For this review, take the finished solid that the model builds, in its own axes (mm). Face numbers are marked on the shaded views. Coordinates: 2 decimals unless noted, no trailing zeros. Loops run counter-clockwise (first coordinate to the right, second up) from the corner with the lowest first, then second, coordinate; pieces in that order, holes last. Notation, with made-up numbers: (67, 68) -> (107, 68) arc R22 cw to (107, 88) -> close; hole circle Ø2 at (-19, 80). An arc over 180 degrees is marked (long way). Answer in a Markdown table with one row per item.
from build123d import *

# Parameters (mm, degrees)
F1_DEPTH = 7.2


with BuildPart() as f1:
    # F0 (on Top) → F1 (new body)
    with BuildSketch(Plane.XY):
        with BuildLine():
            ThreePointArc((-22.7073595632, -1.902869179), (-37.6721050646, -21.75), (-13.0016128307, -18.7137156451))
            ThreePointArc((-13.0016128307, -18.7137156451), (-14.4400957969, -19.1971358452), (-15.9320338179, -19.4747133584))
            ThreePointArc((-15.9320338179, -19.4747133584), (-35.5070415552, -20.5), (-24.8316134088, -4.060189341))
            ThreePointArc((-24.8316134088, -4.060189341), (-23.8452552203, -2.9069218706), (-22.7073595632, -1.902869179))
        make_face()
        with BuildLine():
            ThreePointArc((-6.75, -11.6913429511), (-9.545941546, -9.545941546), (-11.6913429511, -6.75))
            Line((-11.6913429511, -6.75), (-14.2894191624, -8.25))
            ThreePointArc((-14.2894191624, -8.25), (-12.9407634586, -11.5059428911), (-12.4807621135, -15))
            ThreePointArc((-12.4807621135, -15), (-12.6116088995, -16.8750312906), (-13.0016128307, -18.7137156451))
            ThreePointArc((-13.0016128307, -18.7137156451), (-9.0739087263, -15.9164124969), (-6.75, -11.6913429511))
        make_face()
        with BuildLine():
            Line((-14.2894191624, -8.25), (-11.6913429511, -6.75))
            ThreePointArc((-11.6913429511, -6.75), (-13.0399986549, -3.4940571089), (-13.5, 0))
            Line((-13.5, 0), (-18.7587036207, 0))
            ThreePointArc((-18.7587036207, 0), (-20.8303192969, -0.7495522538), (-22.7073595632, -1.902869179))
            ThreePointArc((-22.7073595632, -1.902869179), (-17.8531905577, -4.2207337632), (-14.2894191624, -8.25))
        make_face()
        with BuildLine():
            Line((-16.4544826719, -9.5), (-14.2894191624, -8.25))
            ThreePointArc((-14.2894191624, -8.25), (-17.8531905577, -4.2207337632), (-22.7073595632, -1.902869179))
            ThreePointArc((-22.7073595632, -1.902869179), (-23.8452552203, -2.9069218706), (-24.8316134088, -4.060189341))
            ThreePointArc((-24.8316134088, -4.060189341), (-19.9900128675, -5.7744418342), (-16.4544826719, -9.5))
        make_face()
        with BuildLine():
            ThreePointArc((-12.4807621135, -15), (-12.9407634586, -11.5059428911), (-14.2894191624, -8.25))
            Line((-14.2894191624, -8.25), (-16.4544826719, -9.5))
            ThreePointArc((-16.4544826719, -9.5), (-15.3555780244, -12.1529905039), (-14.9807621135, -15))
            ThreePointArc((-14.9807621135, -15), (-15.221207958, -17.2873553231), (-15.9320338179, -19.4747133584))
            ThreePointArc((-15.9320338179, -19.4747133584), (-14.4400957969, -19.1971358452), (-13.0016128307, -18.7137156451))
            ThreePointArc((-13.0016128307, -18.7137156451), (-12.6116088995, -16.8750312906), (-12.4807621135, -15))
        make_face()
        with BuildLine():
            Line((16.4544826719, -9.5), (14.2894191624, -8.25))
            ThreePointArc((14.2894191624, -8.25), (12.5818579404, -13.35094968), (13.0016128307, -18.7137156451))
            ThreePointArc((13.0016128307, -18.7137156451), (14.4400957969, -19.1971358452), (15.9320338179, -19.4747133584))
            ThreePointArc((15.9320338179, -19.4747133584), (14.9958197548, -14.4246380482), (16.4544826719, -9.5))
        make_face()
        with BuildLine():
            Line((14.2894191624, -8.25), (11.6913429511, -6.75))
            ThreePointArc((11.6913429511, -6.75), (9.545941546, -9.545941546), (6.75, -11.6913429511))
            ThreePointArc((6.75, -11.6913429511), (9.0739087263, -15.9164124969), (13.0016128307, -18.7137156451))
            ThreePointArc((13.0016128307, -18.7137156451), (12.5818579404, -13.35094968), (14.2894191624, -8.25))
        make_face()
        with BuildLine():
            Line((18.7587036207, 0), (13.5, 0))
            ThreePointArc((13.5, 0), (13.0399986549, -3.4940571089), (11.6913429511, -6.75))
            Line((11.6913429511, -6.75), (14.2894191624, -8.25))
            ThreePointArc((14.2894191624, -8.25), (17.8531905577, -4.2207337632), (22.7073595632, -1.902869179))
            ThreePointArc((22.7073595632, -1.902869179), (20.8303192969, -0.7495522538), (18.7587036207, 0))
        make_face()
        with BuildLine():
            ThreePointArc((39.4807621135, -15), (34.2891634511, -4.3594893349), (22.7073595632, -1.902869179))
            ThreePointArc((22.7073595632, -1.902869179), (23.8452552203, -2.9069218706), (24.8316134088, -4.060189341))
            ThreePointArc((24.8316134088, -4.060189341), (33.3414470086, -6.8256304294), (36.9807621135, -15))
            ThreePointArc((36.9807621135, -15), (28.2681174366, -25.7595541555), (15.9320338179, -19.4747133584))
            ThreePointArc((15.9320338179, -19.4747133584), (14.4400957969, -19.1971358452), (13.0016128307, -18.7137156451))
            ThreePointArc((13.0016128307, -18.7137156451), (27.8557934041, -28.369153214), (39.4807621135, -15))
        make_face()
        with BuildLine():
            ThreePointArc((22.7073595632, -1.902869179), (17.8531905577, -4.2207337632), (14.2894191624, -8.25))
            Line((14.2894191624, -8.25), (16.4544826719, -9.5))
            ThreePointArc((16.4544826719, -9.5), (19.9900128675, -5.7744418342), (24.8316134088, -4.060189341))
            ThreePointArc((24.8316134088, -4.060189341), (23.8452552203, -2.9069218706), (22.7073595632, -1.902869179))
        make_face()
        with BuildLine():
            ThreePointArc((0, 11), (5.5, 9.5262794416), (9.5262794416, 5.5))
            Line((9.5262794416, 5.5), (11.6913429511, 6.75))
            ThreePointArc((11.6913429511, 6.75), (9.545941546, 9.545941546), (6.75, 11.6913429511))
            ThreePointArc((6.75, 11.6913429511), (3.4940571089, 13.0399986549), (0, 13.5))
            Line((0, 13.5), (0, 11))
        make_face()
        with BuildLine():
            ThreePointArc((9.5262794416, 5.5), (10.6251840892, 2.8470094961), (11, 0))
            Line((11, 0), (13.5, 0))
            ThreePointArc((13.5, 0), (13.0399986549, 3.4940571089), (11.6913429511, 6.75))
            Line((11.6913429511, 6.75), (9.5262794416, 5.5))
        make_face()
        with BuildLine():
            Line((13.5, 0), (11, 0))
            ThreePointArc((11, 0), (10.6251840892, -2.8470094961), (9.5262794416, -5.5))
            Line((9.5262794416, -5.5), (11.6913429511, -6.75))
            ThreePointArc((11.6913429511, -6.75), (13.0399986549, -3.4940571089), (13.5, 0))
        make_face()
        with BuildLine():
            Line((11.6913429511, -6.75), (9.5262794416, -5.5))
            ThreePointArc((9.5262794416, -5.5), (5.5, -9.5262794416), (0, -11))
            Line((0, -11), (0, -13.5))
            ThreePointArc((0, -13.5), (3.4940571089, -13.0399986549), (6.75, -11.6913429511))
            ThreePointArc((6.75, -11.6913429511), (9.545941546, -9.545941546), (11.6913429511, -6.75))
        make_face()
        with BuildLine():
            Line((0, -13.5), (0, -11))
            ThreePointArc((0, -11), (-5.5, -9.5262794416), (-9.5262794416, -5.5))
            Line((-9.5262794416, -5.5), (-11.6913429511, -6.75))
            ThreePointArc((-11.6913429511, -6.75), (-9.545941546, -9.545941546), (-6.75, -11.6913429511))
            ThreePointArc((-6.75, -11.6913429511), (-3.4940571089, -13.0399986549), (0, -13.5))
        make_face()
        with BuildLine():
            Line((-11.6913429511, -6.75), (-9.5262794416, -5.5))
            ThreePointArc((-9.5262794416, -5.5), (-10.6251840892, -2.8470094961), (-11, 0))
            Line((-11, 0), (-13.5, 0))
            ThreePointArc((-13.5, 0), (-13.0399986549, -3.4940571089), (-11.6913429511, -6.75))
        make_face()
        with BuildLine():
            Line((-13.5, 0), (-11, 0))
            ThreePointArc((-11, 0), (-10.6251840892, 2.8470094961), (-9.5262794416, 5.5))
            Line((-9.5262794416, 5.5), (-11.6913429511, 6.75))
            ThreePointArc((-11.6913429511, 6.75), (-13.0399986549, 3.4940571089), (-13.5, 0))
        make_face()
        with BuildLine():
            ThreePointArc((-9.5262794416, 5.5), (-5.5, 9.5262794416), (0, 11))
            Line((0, 11), (0, 13.5))
            ThreePointArc((0, 13.5), (-3.4940571089, 13.0399986549), (-6.75, 11.6913429511))
            ThreePointArc((-6.75, 11.6913429511), (-9.545941546, 9.545941546), (-11.6913429511, 6.75))
            Line((-11.6913429511, 6.75), (-9.5262794416, 5.5))
        make_face()
        with BuildLine():
            ThreePointArc((-6.75, 11.6913429511), (-3.4940571089, 13.0399986549), (0, 13.5))
            Line((0, 13.5), (0, 16.5))
            ThreePointArc((0, 16.5), (-5.2713326173, 17.5716834431), (-9.7057467326, 20.6165848241))
            ThreePointArc((-9.7057467326, 20.6165848241), (-9.2470631962, 15.816441717), (-6.75, 11.6913429511))
        make_face()
        with BuildLine():
            Line((0, 16.5), (0, 13.5))
            ThreePointArc((0, 13.5), (3.4940571089, 13.0399986549), (6.75, 11.6913429511))
            ThreePointArc((6.75, 11.6913429511), (9.2470631962, 15.816441717), (9.7057467326, 20.6165848241))
            ThreePointArc((9.7057467326, 20.6165848241), (5.2713326173, 17.5716834431), (0, 16.5))
        make_face()
        with BuildLine():
            Line((0, 19), (0, 16.5))
            ThreePointArc((0, 16.5), (5.2713326173, 17.5716834431), (9.7057467326, 20.6165848241))
            ThreePointArc((9.7057467326, 20.6165848241), (9.4051594234, 22.1040577159), (8.8995795909, 23.5349026995))
            ThreePointArc((8.8995795909, 23.5349026995), (4.9941931127, 20.1990798823), (0, 19))
        make_face()
        with BuildLine():
            ThreePointArc((-9.7057467326, 20.6165848241), (-5.2713326173, 17.5716834431), (0, 16.5))
            Line((0, 16.5), (0, 19))
            ThreePointArc((0, 19), (-4.9941931127, 20.1990798823), (-8.8995795909, 23.5349026995))
            ThreePointArc((-8.8995795909, 23.5349026995), (-9.4051594234, 22.1040577159), (-9.7057467326, 20.6165848241))
        make_face()
        with BuildLine():
            ThreePointArc((8.8995795909, 23.5349026995), (9.4051594234, 22.1040577159), (9.7057467326, 20.6165848241))
            ThreePointArc((9.7057467326, 20.6165848241), (12.5155419557, 24.9392481235), (13.5, 30))
            ThreePointArc((13.5, 30), (-5.0607518765, 42.5155419557), (-9.7057467326, 20.6165848241))
            ThreePointArc((-9.7057467326, 20.6165848241), (-9.4051594234, 22.1040577159), (-8.8995795909, 23.5349026995))
            ThreePointArc((-8.8995795909, 23.5349026995), (-3.3988692605, 40.4617248936), (11, 30))
            ThreePointArc((11, 30), (10.4617248936, 26.6011307395), (8.8995795909, 23.5349026995))
        make_face()
    extrude(amount=F1_DEPTH)


solid = f1.part
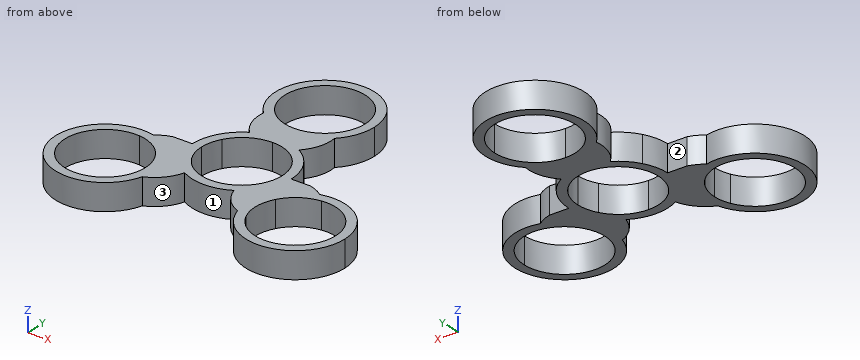
Item 1: For L1, parallel to Y at x = -0.5, z = 1.25; L2, parallel to X at y = 30, z = 4.5; L3, parallel to Y at x = -8.5, z = 2.5, list the stretches that pass through material, from the lowest coordinate up.
Worked answers:
| item | result |
|---|---|
| L1 | -13.49 to -10.99, 10.99 to 19.01, 40.99 to 43.49 |
| L2 | -13.5 to -11, 11 to 13.5 |
| L3 | -15.21 to -6.98, 6.98 to 10.49, 14.08 to 23.02, 36.98 to 40.49 |
Item 2: Insertion check: pin 1 (4 mm diameter, centred on x = -16.5, z = 2.5, fed in from +Y); pin 2 (3 mm diameter, centred on y = 3, z = 6.5, fed in from -X); pin 3 (4 mm diameter, centred on y = 8.5, z = 3.5, fed in from +X); pin 4 (1.5 mm diameter, centred on x = 19, y = -20, fed in from +Z). Each pin has a flat end and moves straight along its axis. Give the tip position at first contact, or say it passes through.
Worked answers:
| item | result |
|---|---|
| pin 1 | y = 0 |
| pin 2 | x = -13.42 |
| pin 3 | x = 11.83 |
| pin 4 | through |
Item 3: Take a section at B-B, the plane x = -31. State the section outline as (y, z) points, and give its area (3 significant figures).
Worked answers:
| item | result |
|---|---|
| outline | (-27.53, 0) -> (-24.79, 0) -> (-24.79, 7.2) -> (-27.53, 7.2) -> close; (-5.21, 0) -> (-2.47, 0) -> (-2.47, 7.2) -> (-5.21, 7.2) -> close |
| area | 39.5 mm² |
Item 4: Take a section at A-A, the plane y = 3.5. State the section outline as (x, z) points, and give its area (3 significant figures).
Worked answers:
| item | result |
|---|---|
| outline | (-13.04, 0) -> (-10.43, 0) -> (-10.43, 7.2) -> (-13.04, 7.2) -> close; (10.43, 0) -> (13.04, 0) -> (13.04, 7.2) -> (10.43, 7.2) -> close |
| area | 37.6 mm² |
Item 5: Take a section at C-C, the plane x = 5. State the section outline as (y, z) points, and give its area (3 significant figures).
Worked answers:
| item | result |
|---|---|
| outline | (-12.54, 0) -> (-9.8, 0) -> (-9.8, 7.2) -> (-12.54, 7.2) -> close; (9.8, 0) -> (20.2, 0) -> (20.2, 7.2) -> (9.8, 7.2) -> close; (39.8, 0) -> (42.54, 0) -> (42.54, 7.2) -> (39.8, 7.2) -> close |
| area | 114 mm² |
Item 6: The part is to be moulded in two halves that separate along X. For the marked faces 1, 2 and 3, say which applies: +X half, -X half, draft (parallel to the pull), parting line (faces both ways), or undercut.
Worked answers:
| item | result |
|---|---|
| face 1 | undercut |
| face 2 | draft |
| face 3 | undercut |
Item 7: Take a section at D-D, the plane x = -3.5. State the section outline as (y, z) points, and give its area (3 significant figures).
Worked answers:
| item | result |
|---|---|
| outline | (-13.04, 0) -> (-10.43, 0) -> (-10.43, 7.2) -> (-13.04, 7.2) -> close; (10.43, 0) -> (19.57, 0) -> (19.57, 7.2) -> (10.43, 7.2) -> close; (40.43, 0) -> (43.04, 0) -> (43.04, 7.2) -> (40.43, 7.2) -> close |
| area | 103 mm² |
